Build history of the part. All positions in model axes, mm. A direction names the side the tool comes from. Give positions to 0.01 mm unless a question says otherwise; leave off trailing zeros. Loops run counter-clockwise (first coordinate to the right, second up) from the corner with the lowest first, then second, coordinate; pieces in that order, holes last. Notation, with made-up numbers: (55, 61.5) -> (98, 61.5) arc R18 ccw to (98, 77.5) -> close; hole circle Ø3 at (53.25, 13.5). An arc over 180 degrees is marked (long way). Answer in a Markdown table with one row per item. Add a question column.
from build123d import *

# Parameters (mm, degrees)
F1_DEPTH  = 30
F3_D      = 3.2
F4_R      = 4
F4_W      = 3.5
F4_H      = 10
F5_DEPTH  = 35.001
F6_SIZE   = 1
F7_R      = 2
F8_R      = 4
F10_DEPTH = 6.001


with BuildPart() as f1:
    # F0 (on Right) → F1 (new body, symmetric)
    with BuildSketch(Plane.YZ):
        Polygon((-17.5, 0), (17.5, 0), (17.5, 30), (11.5, 30), (11.5, 6), (-17.5, 6), align=None)
    extrude(amount=F1_DEPTH, both=True)

    # F3 (through all)
    with Locations(Plane.XY.offset(6)):
        with Locations((-21.5, -2.5), (21.5, -2.5)):
            Hole(F3_D / 2)

    # F4 (on face) → F5 (cut, through all)
    with BuildSketch(Plane(origin=(0, 17.5, 0), x_dir=(-1, 0, 0), z_dir=(0, 1, 0))):
        with Locations((-15, 15)):
            Circle(F4_R)
        with Locations((15, 15)):
            Circle(F4_R)
        with Locations((28.25, 15)):
            Rectangle(F4_W, F4_H)
        with Locations((-28.25, 15)):
            Rectangle(F4_W, F4_H)
    extrude(amount=-F5_DEPTH, mode=Mode.SUBTRACT)

    # F6
    f6_edges = [f1.edges().sort_by_distance(p)[0] for p in [
        (-30, 14.5, 20),
        (-30, 14.5, 10),
        (30, 14.5, 20),
        (30, 14.5, 10),
    ]]
    chamfer(f6_edges, length=F6_SIZE)

    # F7
    f7_edges = [f1.edges().sort_by_distance(p)[0] for p in [
        (-30, 14.5, 30),
        (30, 14.5, 30),
    ]]
    fillet(f7_edges, radius=F7_R)

    # F8
    f8_edges = [f1.edges().sort_by_distance(p)[0] for p in [
        (-30, -17.5, 3),
        (30, -17.5, 3),
    ]]
    fillet(f8_edges, radius=F8_R)

    # F9 (on face) → F10 (cut, through all)
    with BuildSketch(Plane.XY.offset(6)):
        with BuildLine():
            ThreePointArc((2.5, 5), (0, 7.5), (-2.5, 5))
            Line((-2.5, 5), (-2.5, -10))
            ThreePointArc((-2.5, -10), (0, -12.5), (2.5, -10))
            Line((2.5, -10), (2.5, 5))
        make_face()
    extrude(amount=-F10_DEPTH, mode=Mode.SUBTRACT)


solid = f1.part
(1) Saw through at C-C, the plane y = 3.5. List the corners of the cut face in (x, z).
(2) 3-axis set-ups, long thin cutter, end or side, ignore diameter. For faces 1 (the flat face through (0, 11.5, 18)), 2 (the cylindrical face through (-0.1, -12.5, 3)), 3 (the flat face through (-30, 14, 25)), 4 (the flat face through (-28, 15, 10)): which of +Z, -Z, +X, -X, +Y, -Y reach the whole face in a straight line?
(3) Saw through at D-D, the plane z = 17.75. List the corners of the cut face in (x, y), then the cut area to 3 significant figures.
(4) Two-plate mould, pull along Z, no slides. Class faces 5 (the flat face through (30, 2, 4)), 6 (the flat face through (0, 15, 30)), 7 (the flat face through (26.5, 15, 15)): released by +Z, released by -Z, zero draft, split by the parting line, or undercut.
(5) Saw through at B-B, the plane y = 12.5. List the corners of the cut face in (x, z).
(6) Wall check: line 1 along Y through (x, z) = (-21.5, 4.1); line 2 along Z through (x, y) = (15, 13); line 3 along Z through (x, y) = (10.5, -2). Give the ranges that are in metal, low to high. Write a range as from..to.
(7) Flat gauge pins, fed straight in: pin 1 Ø5 at (y, z) = (14.5, 13.5) entering from +X; pin 2 Ø12 at (x, z) = (-18.5, 26.5) entering from -Y; pin 3 Ø1 at (x, y) = (-4, 2.5) entering from +Z. Where does each tip first touch, or does it go through?
(8) Saw through at A-A, the plane x = 0. List the corners of the cut face in (y, z).
Worked answers:
| question | item | result |
|---|---|---|
| 1 | outline | (-30, 0) -> (-2.5, 0) -> (-2.5, 6) -> (-30, 6) -> close; (2.5, 0) -> (30, 0) -> (30, 6) -> (2.5, 6) -> close |
| 2 | face 1 | +Z, +X, -X, -Y |
| 2 | face 2 | +Z, -Z |
| 2 | face 3 | +Z, -Z, -X, +Y, -Y |
| 2 | face 4 | -X, +Y, -Y |
| 3 | outline | (-26.5, 11.5) -> (-17.9, 11.5) -> (-17.9, 17.5) -> (-26.5, 17.5) -> close; (-12.1, 11.5) -> (12.1, 11.5) -> (12.1, 17.5) -> (-12.1, 17.5) -> close; (17.9, 11.5) -> (26.5, 11.5) -> (26.5, 17.5) -> (17.9, 17.5) -> close |
| 3 | area | 248 mm^2 |
| 4 | face 5 | zero draft |
| 4 | face 6 | released by +Z |
| 4 | face 7 | undercut |
| 5 | outline | (-30, 0) -> (30, 0) -> (30, 9) -> (29, 10) -> (26.5, 10) -> (26.5, 20) -> (29, 20) -> (30, 21) -> (30, 28) arc R2 ccw to (28, 30) -> (-28, 30) arc R2 ccw to (-30, 28) -> (-30, 21) -> (-29, 20) -> (-26.5, 20) -> (-26.5, 10) -> (-29, 10) -> (-30, 9) -> close; hole circle Ø8 at (-15, 15); hole circle Ø8 at (15, 15) |
| 6 | line 1 | -17.5..-4.1, -0.9..17.5 |
| 6 | line 2 | 0..11, 19..30 |
| 6 | line 3 | 0..6 |
| 7 | pin 1 | x = 26.5 |
| 7 | pin 2 | y = 11.5 |
| 7 | pin 3 | z = 6 |
| 8 | outline | (-17.5, 0) -> (-12.5, 0) -> (-12.5, 6) -> (-17.5, 6) -> close; (7.5, 0) -> (17.5, 0) -> (17.5, 30) -> (11.5, 30) -> (11.5, 6) -> (7.5, 6) -> close |
